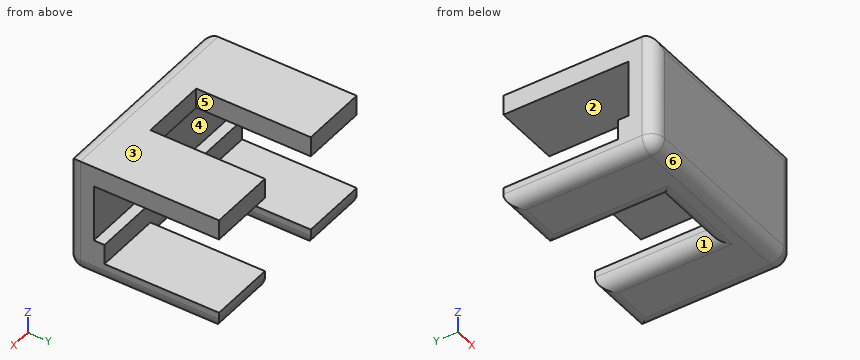
from build123d import *

# Parameters (mm, degrees)
SKETCH1_W           = 30
SKETCH1_H           = 17.5
BOSS_EXTRUDE1_DEPTH = 4
SKETCH2_W           = 30
SKETCH2_H           = 6
BOSS_EXTRUDE2_DEPTH = 1.601
SKETCH3_W           = 10
SKETCH3_H           = 3
BOSS_EXTRUDE3_DEPTH = 18.7
SKETCH4_W           = 10
SKETCH4_H           = 3
BOSS_EXTRUDE4_DEPTH = 17.099
SKETCH5_W           = 10
SKETCH5_H           = 3
BOSS_EXTRUDE5_DEPTH = 1.601
FILLET1_R           = 2


with BuildPart() as part:
    # Sketch1 → Boss-Extrude1 (new body)
    with BuildSketch(Plane(origin=(0, 0, 0), x_dir=(1, 0, 0), z_dir=(0, 1, 0))):
        with Locations((15, 8.75)):
            Rectangle(SKETCH1_W, SKETCH1_H)
    extrude(amount=BOSS_EXTRUDE1_DEPTH)

    # Sketch2 → Boss-Extrude2 (add)
    with BuildSketch(Plane(origin=(0, 4, 0), x_dir=(1, 0, 0), z_dir=(0, 1, 0))):
        with Locations((15, 14.5)):
            Rectangle(SKETCH2_W, SKETCH2_H)
    extrude(amount=BOSS_EXTRUDE2_DEPTH)

    # Sketch3 → Boss-Extrude3 (add)
    with BuildSketch(Plane(origin=(0, 4, 0), x_dir=(1, 0, 0), z_dir=(0, 1, 0))):
        with Locations((5, 1.5)):
            Rectangle(SKETCH3_W, SKETCH3_H)
        with Locations((25, 1.5)):
            Rectangle(SKETCH3_W, SKETCH3_H)
    extrude(amount=BOSS_EXTRUDE3_DEPTH)

    # Sketch4 → Boss-Extrude4 (add)
    with BuildSketch(Plane(origin=(0, 5.601, 0), x_dir=(1, 0, 0), z_dir=(0, 1, 0))):
        with Locations((5, 16)):
            Rectangle(SKETCH4_W, SKETCH4_H)
        with Locations((25, 16)):
            Rectangle(SKETCH4_W, SKETCH4_H)
    extrude(amount=BOSS_EXTRUDE4_DEPTH)

    # Sketch5 → Boss-Extrude5 (add)
    with BuildSketch(Plane(origin=(0, 4, 0), x_dir=(1, 0, 0), z_dir=(0, 1, 0))):
        with Locations((15, 1.5)):
            Rectangle(SKETCH5_W, SKETCH5_H)
    extrude(amount=BOSS_EXTRUDE5_DEPTH)

    # Fillet1
    fillet1_edges = [part.edges().sort_by_distance(p)[0] for p in [
        (15, 0, -17.5),
        (30, 0, -8.75),
        (15, 0, 0),
        (10, 14.1505, -17.5),
        (5, 22.7, -17.5),
        (0, 0, -8.75),
        (15, 5.601, -17.5),
        (20, 14.1505, -17.5),
        (25, 22.7, -17.5),
        (0, 11.35, -17.5),
        (30, 11.35, -17.5),
    ]]
    fillet(fillet1_edges, radius=FILLET1_R)


solid = part.part
Can you work these out from the model? Positions are in its coordinate system, mm. Face numbers are marked on the shaded views. A direction names the side the tool comes from. Give positions to 0.01 mm unless a question says otherwise; leave off trailing zeros. Loops run counter-clockwise (first coordinate to the right, second up) from the corner with the lowest first, then second, coordinate; pieces in that order, holes last. Notation, with made-up numbers: M -29.5,37 L -7.5,37 A17 cw -7.5,55 Z; hole C -18,62.5 d5. An arc over 180 degrees is marked long. One line per item, written item: value. Start each with the question number.
1) Thinking about a two-plate mould opening in Z: for the marked faces 4, 5 and 6, which applies, +Z half, -Z half, draft (parallel to the pull), parting line (faces both ways), or undercut?
2) If we section it at D-D, the plane y = 5: Write out the boundary of the cut face in (x, z), and give its area (3 significant figures).
3) I'm going to push a flat-ended pin straight in: pin 1 (2.5 mm diameter, centred on x = 13.5, z = -1, fed in from +Y). Where does the tip first touch, or does it pass through?
4) If we section it at B-B, the plane z = -2.5: Write out the boundary of the cut face in (x, y), and give its area (3 significant figures).
5) If we section it at A-A, the plane y = 15.5: Write out the boundary of the cut face in (x, z).
6) If I drill on line 1 (Z direction, x = 4.75, y = 20.5); line 2 (Y direction, x = 15, z = -7); line 3 (Z direction, x = 9, y = 15.25), over which ranges is the centre line in solid material (lowest first)? Write a range as [from, to].
7) If we section it at C-C, the plane x = 27.5: Write out the boundary of the cut face in (y, z), and give its area (3 significant figures).
8) On a 3-axis mill with a long thin cutter (end or side, diameter ignored), from which of +Z, -Z, +X, -X, +Y, -Y can I reach the whole of each face in a straight line? I mean the marked faces 1, 2 and 3. Say none if no direction works.
Completed:
1. face 4: undercut
1. face 5: draft
1. face 6: -Z half
2. outline: M 0,-15.5 A2 ccw 2,-17.5 L 8,-17.5 A2 ccw 9.4,-16.93 L 20.6,-16.93 A2 ccw 22,-17.5 L 28,-17.5 A2 ccw 30,-15.5 L 30,-11.5 L 0,-11.5 Z; M 0,-3 L 30,-3 L 30,0 L 0,0 Z
2. area: 261 mm^2
3. pin 1: stops at y = 5.6
4. outline: M 0,2 A2 ccw 2,0 L 28,0 A2 ccw 30,2 L 30,22.7 L 20,22.7 L 20,5.6 L 10,5.6 L 10,22.7 L 0,22.7 Z
4. area: 508 mm^2
5. outline: M 0,-15.5 A2 ccw 2,-17.5 L 8,-17.5 A2 ccw 10,-15.5 L 10,-14.5 L 0,-14.5 Z; M 0,-3 L 10,-3 L 10,0 L 0,0 Z; M 20,-15.5 A2 ccw 22,-17.5 L 28,-17.5 A2 ccw 30,-15.5 L 30,-14.5 L 20,-14.5 Z; M 20,-3 L 30,-3 L 30,0 L 20,0 Z
6. line 1: z = [-17.5, -14.5], [-3, 0]
6. line 2: y = [0, 4]
6. line 3: z = [-17.23, -14.5], [-3, 0]
7. outline: M 0,-15.5 A2 ccw 2,-17.5 L 20.7,-17.5 A2 ccw 22.7,-15.5 L 22.7,-14.5 L 5.6,-14.5 L 5.6,-11.5 L 4,-11.5 L 4,-3 L 22.7,-3 L 22.7,0 L 2,0 A2 ccw 0,-2 Z
7. area: 184 mm^2
8. face 1: -Z, +Y
8. face 2: +X, -X, +Y
8. face 3: +Z, +X, -X, +Y, -Y
